Verification items for the finished model (mm, model axes). Face numbers are marked on the shaded views. Round coordinates to 2 decimals unless told otherwise and drop trailing zeros. Write each loop counter-clockwise with the first axis right and the second up, starting at its lowest first coordinate (ties: lowest second). Pieces come first, ordered by that corner, then holes.
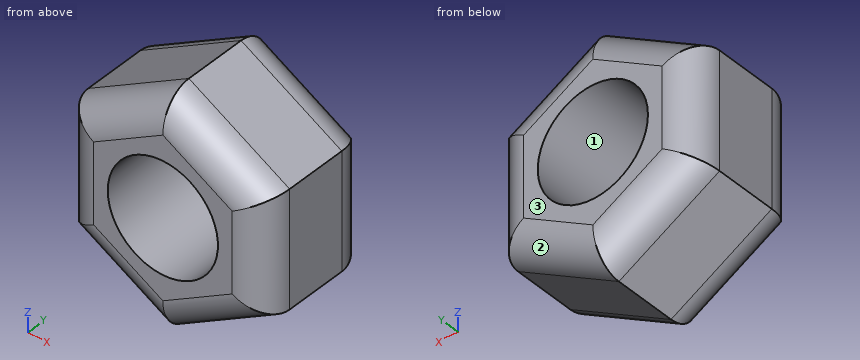
Autodesk Inventor part; units mm, degrees
ref_plane "YZ Plane" through (0, 0, 0) normal (1, 0, 0) x (0, 1, 0)
ref_plane "XZ Plane" through (0, 0, 0) normal (0, 1, 0) x (-1, 0, 0)
ref_plane "XY Plane" through (0, 0, 0) normal (0, 0, 1) x (1, 0, 0)
sketch "Boceto1" plane through (0, 0, 0) normal (0, 1, 0) x (-1, 0, 0)
  line L0 (0, -7.3901) -> (-6.4, -3.695)
  line L1 (-6.4, -3.695) -> (-6.4, 3.695)
  line L2 (-6.4, 3.695) -> (0, 7.3901)
  line L3 (0, 7.3901) -> (6.4, 3.695)
  line L4 (6.4, 3.695) -> (6.4, -3.695)
  line L5 (6.4, -3.695) -> (0, -7.3901)
  circle A0 centre (0, 0) radius 3.5
  dimension "d0" = 6.4
  dimension "d1" = 0
  dimension "d2" = 7
extrude "Extrusión1" add sketch "Boceto1" along normal blind 8
fillet "Empalme1" radius 2 12 edges at (3.2, 8, 5.5426) (-3.2, 8, 5.5426) (-3.2, 8, -5.5426) (3.2, 8, -5.5426) (6.4, 8, 0) (-6.4, 8, 0) (3.2, 0, 5.5426) (6.4, 0, 0) (-3.2, 0, 5.5426) (3.2, 0, -5.5426) (-3.2, 0, -5.5426) (-6.4, 0, 0)
thread "Rosca1"
properties part number "BASE_TUERCA"
Q1. Sectioned sample at C-C (y = 6.5). Enter the section's corners in (x, z).
Recorded:
outline: (-6.34, -3.66) - (0, -7.32) - (6.34, -3.66) - (6.34, 3.66) - (0, 7.32) - (-6.34, 3.66) - close; hole circle Ø7 at (0, 0)
Q2. Sectioned sample at D-D (z = 2.25). Enter the section's corners in (x, y), plus the area to 3 significant figures.
Recorded:
outline: (-6.4, 2) arc R2 ccw to (-4.4, 0) - (-2.68, 0) - (-2.68, 8) - (-4.4, 8) arc R2 ccw to (-6.4, 6) - close; (2.68, 0) - (4.4, 0) arc R2 ccw to (6.4, 2) - (6.4, 6) arc R2 ccw to (4.4, 8) - (2.68, 8) - close
area: 56.1 mm2
Q3. Sectioned sample at A-A (z = 0). Enter the section's corners in (x, y).
Recorded:
outline: (-6.4, 2) arc R2 ccw to (-4.4, 0) - (-3.5, 0) - (-3.5, 8) - (-4.4, 8) arc R2 ccw to (-6.4, 6) - close; (3.5, 0) - (4.4, 0) arc R2 ccw to (6.4, 2) - (6.4, 6) arc R2 ccw to (4.4, 8) - (3.5, 8) - close
Q4. Depth check by flat-ended pin: P1, Ø2, axis at x = -2.5, y = 6, coming from the -Z side; P2, Ø4, axis at x = -2, z = -2, coming from the -Y side; P3, Ø4, axis at x = 0, z = 0, coming from the +Y side. Enter the tip coordinate at first touch or a pass-through.
Recorded:
P1: stops at z = -6.52
P2: stops at y = 0
P3: passes through
Q5. Material ranges on line 1 along Z through (x, y) = (-3, 1.5); line 2 along Z through (x, y) = (-1, 4); line 3 along X through (y, z) = (6.5, 0.5), recorded low to high.
Recorded:
line 1: z = -5.58 to -1.8, 1.8 to 5.58
line 2: z = -6.81 to -3.35, 3.35 to 6.81
line 3: x = -6.34 to -3.46, 3.46 to 6.34
Q6. Sectioned sample at B-B (y = 3.5). Enter the section's corners in (x, z) (3 decimals), plus the area to 3 significant figures.
Recorded:
outline: (-6.4, -3.695) - (0, -7.39) - (6.4, -3.695) - (6.4, 3.695) - (0, 7.39) - (-6.4, 3.695) - close; hole circle Ø7 at (0, 0)
area: 103 mm2
Q7. Release check for a two-part mould opening along Z. For the marked faces 1, 2 and 3 record: released by +Z, released by -Z, zero draft, split by the parting line, or undercut.
Recorded:
face 1: undercut
face 2: released by -Z
face 3: zero draft
